Geometry: final body of the model. Coordinates: model frame, mm. Face numbers are marked on the shaded views. A direction names the side the tool comes from. Coordinates: 2 decimals unless noted, no trailing zeros. Order: outer loops, then holes, each group sorted by start corner. A loop starts at its lowest first (then second) coordinate and runs counter-clockwise, first axis right, second up. Notation, with made-up numbers: M 32.5,-29.75 L 80.5,-29.75 A7 ccw 80.5,-19.75 Z; hole C 71.25,26 d6. An arc over 180 degrees is marked long. One line per question, with ' | ' between items.
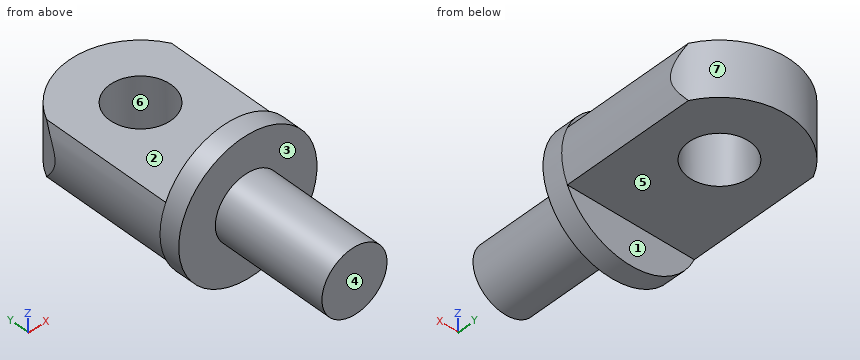
from build123d import *
from build123d.topology import SkipClean

# Parameters (mm, degrees)
SKETCH_1_R          = 3.4
EXTRUDE_3_DEPTH     = 1
EXTRUDE_4_DEPTH     = 8.3
CUT_EXTRUDE_3_DEPTH = 11.982372239
SKETCH_7_R          = 1.5
CUT_EXTRUDE_4_DEPTH = 11.982372355
SKETCH_8_R          = 1.6
EXTRUDE_5_DEPTH     = 5.7


with BuildPart() as part:
    # 草图1 → 凸台-拉伸3 (new body)
    with BuildSketch(Plane(origin=(0, 0, 0), x_dir=(1, 0, 0), z_dir=(0, 1, 0))):
        with Locations(Location((0, 0, 0), (0, 0, 270))):
            Circle(SKETCH_1_R)
    extrude(amount=EXTRUDE_3_DEPTH)

    # 草图5 → 凸台-拉伸4 (add)
    with SkipClean():  # the faces are left unmerged after this step: merging them gives an invalid solid
        with BuildSketch(Plane(origin=(0, 1, 0), x_dir=(1, 0, 0), z_dir=(0, 1, 0))):
            with BuildLine():
                Line((-3.120496755, 1.35), (3.120496755, 1.35))
                ThreePointArc((3.120496755, 1.35), (3.4, 0), (3.120496755, -1.35))
                Line((3.120496755, -1.35), (-3.120496755, -1.35))
                ThreePointArc((-3.120496755, -1.35), (-3.4, 0), (-3.120496755, 1.35))
            make_face()
        extrude(amount=EXTRUDE_4_DEPTH)

    # 草图6 → 切除-拉伸3 (cut, through all)
    with SkipClean():  # the faces are left unmerged after this step: merging them gives an invalid solid
        with BuildSketch(Plane.XY.offset(1.35)):
            with BuildLine():
                Line((-3.4, 6.612575767), (-3.4, 9.766288837))
                Line((-3.4, 9.766288837), (3.4, 9.766288837))
                Line((3.4, 9.766288837), (3.4, 6.81399223))
                ThreePointArc((3.4, 6.81399223), (-0.076572867, 9.298452515), (-3.4, 6.612575767))
            make_face()
        extrude(amount=-CUT_EXTRUDE_3_DEPTH, mode=Mode.SUBTRACT)

    # 草图7 → 切除-拉伸4 (cut, through all)
    with SkipClean():  # the faces are left unmerged after this step: merging them gives an invalid solid
        with BuildSketch(Plane.XY.offset(1.35)):
            with Locations((0.027939034, 5.770037221)):
                Circle(SKETCH_7_R)
        extrude(amount=-CUT_EXTRUDE_4_DEPTH, mode=Mode.SUBTRACT)

    # 草图8 → 凸台-拉伸5 (add)
    with SkipClean():  # the faces are left unmerged after this step: merging them gives an invalid solid
        with BuildSketch(Plane.XZ):
            with Locations(Location((0, 0, 0), (0, 0, 270))):
                Circle(SKETCH_8_R)
        extrude(amount=EXTRUDE_5_DEPTH)


solid = part.part
1. Access query for the marked faces 1, 2 and 3. Directions: +Z, -Z, +X, -X, +Y, -Y. A direction counts if a zero-diameter tool reaches every point of the face in a straight line with its end or side. Return the directions, or none.
Response values:
face 1: -Z, +X, -X, +Y | face 2: +Z, +X, -X, +Y | face 3: -Y
2. Section D-D, the plane x = 1.75. Output: boundary loops of the cut face in (y, z), and give its area (3 significant figures).
Response values:
outline: M 0,-2.92 L 1,-2.92 L 1,-1.35 L 8.85,-1.35 L 8.85,1.35 L 1,1.35 L 1,2.92 L 0,2.92 Z | area: 27.0 mm^2
3. Pin query (flat end, axial travel): P1, Ø2, axis at y = 1, z = 1.5, coming from the +X side; P2, Ø2, axis at x = 2.5, y = 3.5, coming from the -Z side; P3, Ø1.9, axis at x = 1.5, y = 4.5, coming from the +Z side. Return the tip coordinate at first contact, or that it passes through.
Response values:
P1: stops at x = 3.36 | P2: stops at z = -1.35 | P3: stops at z = 1.35
4. Section A-A, the plane x = 0. Output: boundary loops of the cut face in (y, z).
Response values:
outline: M -5.7,-1.6 L 0,-1.6 L 0,-3.4 L 1,-3.4 L 1,-1.35 L 4.27,-1.35 L 4.27,1.35 L 1,1.35 L 1,3.4 L 0,3.4 L 0,1.6 L -5.7,1.6 Z; M 7.27,-1.35 L 9.3,-1.35 L 9.3,1.35 L 7.27,1.35 Z
5. Section C-C, the plane y = -1.25. Output: boundary loops of the cut face in (x, z).
Response values:
outline: C 0,0 d3.2
6. Material intervals for line 1 (Z direction, x = -1, y = 1.5); line 2 (Y direction, x = 1.25, z = 2.25); line 3 (Y direction, x = -0.25, z = -0.5), sorted ascending. Write a range as [from, to].
Response values:
line 1: z = [-1.35, 1.35] | line 2: y = [0, 1] | line 3: y = [-5.7, 4.3], [7.24, 9.29]
7. Section B-B, the plane z = 0. Output: boundary loops of the cut face in (x, y), and give its area (3 significant figures).
Response values:
outline: M -3.4,0 L -1.6,0 L -1.6,-5.7 L 1.6,-5.7 L 1.6,0 L 3.4,0 L 3.4,6.81 A3.53 ccw -3.4,6.61 Z; hole C 0.03,5.77 d3 | area: 69.8 mm^2
8. Draft query along Y for the marked faces 4, 5, 6 and 7. Return one class per face: pulls with the +Y half, pulls with the -Y half, needs draft (parallel to the pull), parting line crosses it, or undercut.
Response values:
face 4: pulls with the -Y half | face 5: needs draft | face 6: undercut | face 7: pulls with the +Y half
